```python
from build123d import *

# Parameters (mm, degrees)
BASE_EXTRUDE_DEPTH   = 285.75
BOSS_EXTRUDE1_DEPTH  = 25.4
FILLET1_R            = 25.4
SKETCH3_R            = 19.05
CUT_EXTRUDE1_DEPTH   = 25.4
FILLET1_OF_MIRROR1_R = 25.4


with BuildPart() as part:
    # Sketch1 → Base-Extrude (new body)
    with BuildSketch(Plane(origin=(0, 0, 0), x_dir=(0, 0, -1), z_dir=(1, 0, 0))):
        with BuildLine():
            Line((-85.725, 0), (-101.6, 0))
            Line((-101.6, 0), (-101.6, 85.725))
            Line((-101.6, 85.725), (-69.85, 85.725))
            Line((-69.85, 85.725), (-69.85, 107.95))
            Line((-69.85, 107.95), (69.85, 107.95))
            Line((69.85, 107.95), (69.85, 85.725))
            Line((69.85, 85.725), (101.6, 85.725))
            Line((101.6, 85.725), (101.6, 0))
            Line((101.6, 0), (85.725, 0))
            ThreePointArc((85.725, 0), (0, 85.725), (-85.725, 0))
        make_face()
    extrude(amount=-BASE_EXTRUDE_DEPTH)

    # Sketch2 → Boss-Extrude1 (add)
    with BuildSketch(Plane.XY.offset(69.85)):
        with BuildLine():
            Line((-180.975, 107.95), (-180.975, 146.05))
            ThreePointArc((-180.975, 146.05), (-142.875, 184.15), (-104.775, 146.05))
            Line((-104.775, 146.05), (-104.775, 107.95))
            Line((-104.775, 107.95), (-180.975, 107.95))
        make_face()
    boss_extrude1 = extrude(amount=-BOSS_EXTRUDE1_DEPTH)

    # Fillet1
    fillet1_edges = [part.edges().sort_by_distance(p)[0] for p in [
        (-104.775, 107.95, 57.15),
        (-180.975, 107.95, 57.15),
    ]]
    fillet(fillet1_edges, radius=FILLET1_R)

    # Sketch3 → Cut-Extrude1 (cut)
    with BuildSketch(Plane.XY.offset(69.85)):
        with Locations((-142.875, 146.05)):
            Circle(SKETCH3_R)
    cut_extrude1 = extrude(amount=-CUT_EXTRUDE1_DEPTH, mode=Mode.SUBTRACT)

    # Mirror1: Boss-Extrude1, Cut-Extrude1 across plane
    add(boss_extrude1.mirror(Plane.XY))
    add(cut_extrude1.mirror(Plane.XY), mode=Mode.SUBTRACT)

    # Fillet1 of Mirror1
    fillet1_of_mirror1_edges = [part.edges().sort_by_distance(p)[0] for p in [
        (-104.775, 107.95, -57.15),
        (-180.975, 107.95, -57.15),
    ]]
    fillet(fillet1_of_mirror1_edges, radius=FILLET1_OF_MIRROR1_R)


solid = part.part
```
Geometry: final body of the model. Coordinates: model frame, mm. A direction names the side the tool comes from. Round coordinates to 2 decimals unless told otherwise and drop trailing zeros. Loops run counter-clockwise (first coordinate to the right, second up) from the corner with the lowest first, then second, coordinate; pieces in that order, holes last.
Item 1: Section A-A, the plane x = -139. Output: boundary loops of the cut face in (y, z) (3 decimals).
Checked values:
outline: (0, -101.6) - (85.725, -101.6) - (85.725, -69.85) - (127.398, -69.85) - (127.398, -44.45) - (107.95, -44.45) - (107.95, 44.45) - (127.398, 44.45) - (127.398, 69.85) - (85.725, 69.85) - (85.725, 101.6) - (0, 101.6) - (0, 85.725) arc R85.725 cw to (0, -85.725) - close; (164.702, -69.85) - (183.952, -69.85) - (183.952, -44.45) - (164.702, -44.45) - close; (164.702, 44.45) - (183.952, 44.45) - (183.952, 69.85) - (164.702, 69.85) - close
Item 2: Section C-C, the plane x = -251. Output: boundary loops of the cut face in (y, z) (3 decimals), plus the area to 3 significant figures.
Checked values:
outline: (0, -101.6) - (85.725, -101.6) - (85.725, -69.85) - (107.95, -69.85) - (107.95, 69.85) - (85.725, 69.85) - (85.725, 101.6) - (0, 101.6) - (0, 85.725) arc R85.725 cw to (0, -85.725) - close
area: 8,980 mm2
Item 3: Section B-B, the plane y = 68. Output: boundary loops of the cut face in (x, z), plus the area to 3 significant figures.
Checked values:
outline: (-285.75, -101.6) - (0, -101.6) - (0, -52.2) - (-285.75, -52.2) - close; (-285.75, 52.2) - (0, 52.2) - (0, 101.6) - (-285.75, 101.6) - close
area: 28,200 mm2
Item 4: Line query: L1, parallel to X at y = 146, z = 58 (3 decimals); L2, parallel to Z at x = -155.5, y = 170; L3, parallel to Y at x = -43, z = 89 (3 decimals). Output: solid intervals per line, ascending.
Checked values:
L1: x = -180.975 to -161.925, -123.825 to -104.775
L2: z = -69.85 to -44.45, 44.45 to 69.85
L3: y = 0 to 85.725
Item 5: Section D-D, the plane y = 142.5. Output: boundary loops of the cut face in (x, z) (3 decimals).
Checked values:
outline: (-180.975, -69.85) - (-161.591, -69.85) - (-161.591, -44.45) - (-180.975, -44.45) - close; (-180.975, 44.45) - (-161.591, 44.45) - (-161.591, 69.85) - (-180.975, 69.85) - close; (-124.159, -69.85) - (-104.775, -69.85) - (-104.775, -44.45) - (-124.159, -44.45) - close; (-124.159, 44.45) - (-104.775, 44.45) - (-104.775, 69.85) - (-124.159, 69.85) - close
Item 6: Contact query for flat-ended pins moving along their axis: P1, Ø10, axis at x = -173.5, z = -38.5, coming from the -Y side; P2, Ø1.5, axis at x = -112.5, y = 145.5, coming from the -Z side; P3, Ø4, axis at y = 138.5, z = -51.5, coming from the +X side (3 decimals). Output: stop coordinate, or through.
Checked values:
P1: stops at y = 73.87
P2: stops at z = -69.85
P3: stops at x = -104.775
Item 7: Reachability of faces 4 (the flat face through (-156, 130, -44.45)), 5 (the flat face through (-104.775, 140, 57)), 6 (the flat face through (-141, 107.95, 1)), 7 (the flat face through (-141, 85.725, -86)), 8 (the flat face through (-141, 112, 69.85)) from +Z, -Z, +X, -X, +Y, -Y: full face, straight path, thin tool, end or side. Return the list, or none.
Checked values:
face 4: +X, -X, +Y
face 5: +Z, -Z, +X, +Y
face 6: +Y
face 7: -Z, +X, -X, +Y
face 8: +Z, +X, -X, +Y
Item 8: Mould query, pull axis X, two halves, no side actions, for faces 1 (the flat face through (-180.975, 140, 57)), 2 (the flat face through (-141, 0, 94)), 3 (the cylindrical face through (-147, 127.45, 57.33)). Classes: released by +X, released by -X, zero draft, split by the parting line, or undercut.
Checked values:
face 1: released by -X
face 2: zero draft
face 3: undercut
